Part model, mm, in its own coordinate system. A direction names the side the tool comes from. Round coordinates to 2 decimals unless told otherwise and drop trailing zeros. Loops run counter-clockwise (first coordinate to the right, second up) from the corner with the lowest first, then second, coordinate; pieces in that order, holes last.
from build123d import *

# Parameters (mm, degrees)
F0_W     = 5
F0_H     = 16.8
F0_W_2   = 10
F0_H_2   = 8.8
F0_W_3   = 15.8
F0_H_3   = 8
F1_DEPTH = 1
F0_H_4   = 2
F2_DEPTH = 2.5
F3_DEPTH = 5
F4_DEPTH = 8
F0_W_4   = 2
F5_DEPTH = 6


with BuildPart() as f1:
    # F0 (on Top) → F1 (new body)
    with BuildSketch(Plane.XY):
        Polygon((69, 24.8), (53.2, 24.8), (53.2, 20.8), (53.2, 16.8), (69, 16.8), align=None)
        Polygon((0, 24.8), (0, 20.8), (6, 20.8), (6, 4), (0, 4), (0, 0), (53.2, 0), (53.2, 8), (53.2, 12.4), (48, 12.4), (48, 20.8), (53.2, 20.8), (53.2, 24.8), align=None)
        with Locations((14.5, 12.4)):
            Rectangle(F0_W, F0_H, mode=Mode.SUBTRACT)
        with Locations((36.3, 12.4)):
            Rectangle(F0_W_2, F0_H_2, mode=Mode.SUBTRACT)
        with Locations((61.1, 4)):
            Rectangle(F0_W_3, F0_H_3)
    extrude(amount=F1_DEPTH)

    # F0 (on Top) → F2 (join)
    with BuildSketch(Plane.XY):
        with Locations((61.1, 25.8)):
            Rectangle(F0_W_3, F0_H_4)
        Polygon((69, 8), (69, 16.8), (53.2, 16.8), (53.2, 12.4), (53.2, 8), align=None)
        with Locations((61.1, -1)):
            Rectangle(F0_W_3, F0_H_4)
        Polygon((69, 26.8), (69, 24.8), (69, 16.8), (69, 8), (69, 0), (69, -2), (71, -2), (71, 26.8), align=None)
    extrude(amount=F2_DEPTH)

    # F0 (on Top) → F3 (join)
    with BuildSketch(Plane.XY):
        Polygon((6, 20.8), (0, 20.8), (0, 16.4), (0, 8.4), (0, 4), (6, 4), align=None)
        with Locations((14.5, 12.4)):
            Rectangle(F0_W, F0_H)
        with Locations((36.3, 12.4)):
            Rectangle(F0_W_2, F0_H_2)
        Polygon((53.2, 16.8), (53.2, 20.8), (48, 20.8), (48, 12.4), (53.2, 12.4), align=None)
    extrude(amount=F3_DEPTH)

    # F0 (on Top) → F4 (join)
    with BuildSketch(Plane.XY):
        Polygon((0, 16.4), (0, 20.8), (0, 24.8), (53.2, 24.8), (53.2, 26.8), (-2, 26.8), (-2, 16.4), align=None)
        Polygon((0, 4), (0, 8.4), (-2, 8.4), (-2, -2), (53.2, -2), (53.2, 0), (0, 0), align=None)
    extrude(amount=F4_DEPTH)

    # F0 (on Top) → F5 (join)
    with BuildSketch(Plane.XY):
        with Locations((-1, 12.4)):
            Rectangle(F0_W_4, F0_H_3)
    extrude(amount=F5_DEPTH)


solid = f1.part
1) Slice it at B-B, the plane y = 3.25. Give the cut face in (x, z).
Values:
outline: (-2, 0) - (71, 0) - (71, 2.5) - (69, 2.5) - (69, 1) - (0, 1) - (0, 8) - (-2, 8) - close
2) Slice it at A-A, the plane z = 4.25. Give the cut face in (x, y).
Values:
outline: (-2, -2) - (53.2, -2) - (53.2, 0) - (0, 0) - (0, 4) - (6, 4) - (6, 20.8) - (0, 20.8) - (0, 24.8) - (53.2, 24.8) - (53.2, 26.8) - (-2, 26.8) - close; (12, 4) - (17, 4) - (17, 20.8) - (12, 20.8) - close; (31.3, 8) - (41.3, 8) - (41.3, 16.8) - (31.3, 16.8) - close; (48, 12.4) - (53.2, 12.4) - (53.2, 20.8) - (48, 20.8) - close
3) Tool access for faces 4 (the face through (51, 17, 5)), 5 (the face through (53.2, 17, 3)), 6 (the face through (21, -1, 8)), 7 (the face through (-1, 8.4, 7)): list every direction of +Z, -Z, +X, -X, +Y, -Y with a clear straight run to the whole face (end or side of a thin tool).
Values:
face 4: +Z, +X
face 5: +Z
face 6: +Z, +X, -X, +Y, -Y
face 7: +Z, +X, -X
4) Slice it at D-D, the plane y = 14. Give the cut face in (x, z), then the cut area to 4 significant figures.
Values:
outline: (-2, 0) - (71, 0) - (71, 2.5) - (53.2, 2.5) - (53.2, 5) - (48, 5) - (48, 1) - (41.3, 1) - (41.3, 5) - (31.3, 5) - (31.3, 1) - (17, 1) - (17, 5) - (12, 5) - (12, 1) - (6, 1) - (6, 5) - (0, 5) - (0, 6) - (-2, 6) - close
area: 214.5 mm2
5) Slice it at C-C, the plane x = 15.5. Give the cut face in (y, z), then the cut area to 3 significant figures.
Values:
outline: (-2, 0) - (26.8, 0) - (26.8, 8) - (24.8, 8) - (24.8, 1) - (20.8, 1) - (20.8, 5) - (4, 5) - (4, 1) - (0, 1) - (0, 8) - (-2, 8) - close
area: 124 mm2
6) Mould opens along Y. For faces 1 (the face through (71, 12, 1)), 2 (the face through (61, 8, 2)), 3 (the face through (27, 26.8, 4)) say: released by +Y, released by -Y, zero draft, split by the parting line, or undercut.
Values:
face 1: zero draft
face 2: undercut
face 3: released by +Y
7) Drop flat-ended pins along their axis: pin 1 Ø1.6 at (y, z) = (25.5, 5) entering from +X; pin 2 Ø7 at (x, y) = (38.5, 13) entering from +Z; pin 3 Ø4 at (x, y) = (58, 13) entering from +Z. Give the stop position or say it passes through.
Values:
pin 1: stops at x = 53.2
pin 2: stops at z = 5
pin 3: stops at z = 2.5
8) Wall check: line 1 along Y through (x, z) = (5, 1.25); line 2 along X through (y, z) = (14.75, 3); line 3 along Y through (x, z) = (9.5, 4.5). Give the ranges that are in metal, low to high.
Values:
line 1: y = -2 to 0, 4 to 20.8, 24.8 to 26.8
line 2: x = -2 to 6, 12 to 17, 31.3 to 41.3, 48 to 53.2
line 3: y = -2 to 0, 24.8 to 26.8
